CAD build for the part. Positions are in the model's coordinates, mm. Give positions to 0.01 mm unless a question says otherwise; leave off trailing zeros. Write each loop counter-clockwise with the first axis right and the second up, starting at its lowest first coordinate (ties: lowest second). Pieces come first, ordered by that corner, then holes. Notation, with made-up numbers: M 31.25,48 L 65.25,48 A20 ccw 65.25,76 Z; hole C -11.75,-25.5 d5. An arc over 180 degrees is marked long. One line per question, with ' | ' between items. Start each with the question number.
1. Flat gauge pins, fed straight in: pin 1 (15 mm diameter, centred on x = 6.5, z = 505.5, fed in from -Y); pin 2 (5 mm diameter, centred on x = 5.5, y = -4, fed in from +Z). Where does each tip first touch, or does it go through?
2. Wall check: L1, parallel to Z at x = 22, y = -1.25; L2, parallel to Z at x = 0, y = -2.75; L3, parallel to X at y = -7.25, z = 247.65. Give the ranges that are in metal, low to high.
3. Cut at A-A, the plane x = 13.5. Write the cut outline in (y, z) (3 decimals), then the cut area to 3 significant figures.
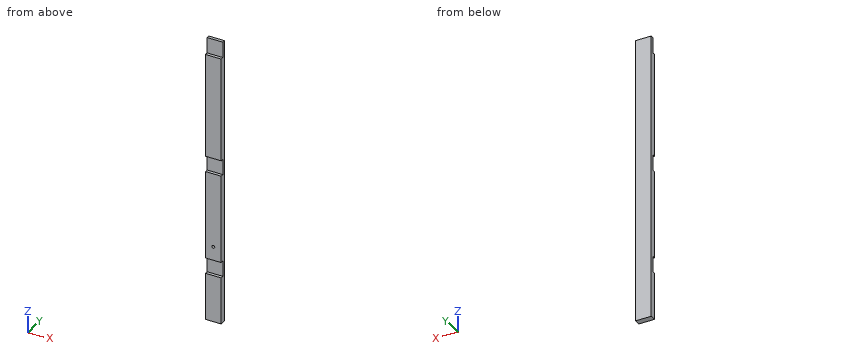
```python
from build123d import *

# Parameters (mm, degrees)
F0_W     = 50.8
F0_H     = 19.05
F1_DEPTH = 927.1
F2_W     = 122.43557321
F2_H     = 50.8
F2_W_2   = 343.1604206562
F2_W_3   = 264.5317912102
F3_DEPTH = 25.4
F4_R     = 4.7625
F5_DEPTH = 25.4


# Not quite as in the source:
# - a feature names something its author has since deleted; it is built from what else it names


with BuildPart() as f1:
    # F0 (on Top) → F1 (new body)
    with BuildSketch(Plane.XY):
        Rectangle(F0_W, F0_H)
    extrude(amount=F1_DEPTH)

    # F2 (on Front) → F3 (cut)
    with BuildSketch(Plane.XZ):
        with Locations((22.4465244144, 177.8)):
            Rectangle(F2_W, F2_H)
        with Locations((-38.7818217278, 901.7)):
            Rectangle(F2_W_2, F2_H)
        with Locations((-47.6498156786, 514.35)):
            Rectangle(F2_W_3, F2_H)
    extrude(amount=F3_DEPTH, mode=Mode.SUBTRACT)

    # F4 (on Front) → F5 (cut)
    with BuildSketch(Plane.XZ):
        with Locations((0, 247.65)):
            Circle(F4_R)
    extrude(amount=F5_DEPTH, mode=Mode.SUBTRACT)


solid = f1.part
```
Here are the results:
1) pin 1: y = 0 | pin 2: z = 876.3
2) L1: 0 to 152.4, 203.2 to 488.95, 539.75 to 876.3 | L2: 0 to 152.4, 203.2 to 242.89, 252.41 to 488.95, 539.75 to 876.3 | L3: -25.4 to -4.76, 4.76 to 25.4
3) outline: M -9.525,0 L 9.525,0 L 9.525,927.1 L 0,927.1 L 0,876.3 L -9.525,876.3 L -9.525,539.75 L 0,539.75 L 0,488.95 L -9.525,488.95 L -9.525,203.2 L 0,203.2 L 0,152.4 L -9.525,152.4 Z | area: 16,200 mm^2
